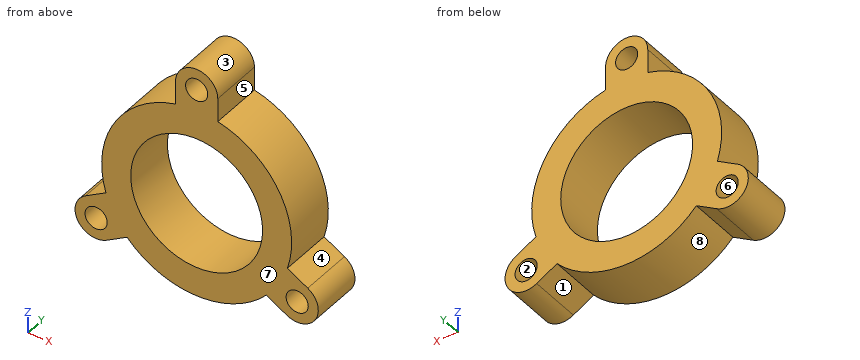
from build123d import *

# Parameters (mm, degrees)
SKETCH1_R           = 2.1
SKETCH1_R_2         = 12.5
BOSS_EXTRUDE1_DEPTH = 10


with BuildPart() as part:
    # Sketch1 → Boss-Extrude1 (new body)
    with BuildSketch(Plane(origin=(0, 0, 0), x_dir=(1, 0, 0), z_dir=(0, 1, 0))):
        with BuildLine():
            ThreePointArc((-4, -22), (0, -26), (4, -22))
            Line((4, -22), (4, -17.549928775))
            ThreePointArc((4, -17.549928775), (15.588457268, -9), (17.198684154, 5.310862772))
            Line((17.198684154, 5.310862772), (21.052558883, 7.535898385))
            ThreePointArc((21.052558883, 7.535898385), (22.516660498, 13), (17.052558883, 14.464101615))
            Line((17.052558883, 14.464101615), (13.198684154, 12.239066003))
            ThreePointArc((13.198684154, 12.239066003), (0, 18), (-13.198684154, 12.239066003))
            Line((-13.198684154, 12.239066003), (-17.052558883, 14.464101615))
            ThreePointArc((-17.052558883, 14.464101615), (-22.516660498, 13), (-21.052558883, 7.535898385))
            Line((-21.052558883, 7.535898385), (-17.198684154, 5.310862772))
            ThreePointArc((-17.198684154, 5.310862772), (-15.588457268, -9), (-4, -17.549928775))
            Line((-4, -17.549928775), (-4, -22))
        make_face()
        with Locations((0, -22)):
            Circle(SKETCH1_R, mode=Mode.SUBTRACT)
        Circle(SKETCH1_R_2, mode=Mode.SUBTRACT)
        with Locations((19.052558883, 11)):
            Circle(SKETCH1_R, mode=Mode.SUBTRACT)
        with Locations((-19.052558883, 11)):
            Circle(SKETCH1_R, mode=Mode.SUBTRACT)
    extrude(amount=BOSS_EXTRUDE1_DEPTH)


solid = part.part
Geometry: final body of the model. Coordinates: model frame, mm. Face numbers are marked on the shaded views. A direction names the side the tool comes from. Give positions to 0.01 mm unless a question says otherwise; leave off trailing zeros. Write each loop counter-clockwise with the first axis right and the second up, starting at its lowest first coordinate (ties: lowest second). Pieces come first, ordered by that corner, then holes. Notation, with made-up numbers: M -15,19.5 L 40,19.5 A17 cw 40,30.5 Z; hole C 34.25,-18.75 d5. An arc over 180 degrees is marked long. Answer in a Markdown table with one row per item. Add a question column.
(1) Ray query, line 1 (Z direction, x = 0, y = 6.5); line 2 (X direction, y = 5.75, z = -0.5); line 3 (X direction, y = 5.75, z = -11). Return the intervals inside material, ascending.
(2) First-contact query: pin 1 (5 mm diameter, centred on y = 2, z = 14, fed in from -X); pin 2 (5 mm diameter, centred on x = 18, y = 5, fed in from +Z); pin 3 (5 mm diameter, centred on y = 5.5, z = 10.5, fed in from -X). Flat tips, straight axial feed; report the tip coordinate or a pass-through.
(3) Reachability of the marked faces 1, 2, 3, 4 and 5 from +Z, -Z, +X, -X, +Y, -Y: full face, straight path, thin tool, end or side. Return the list, or none.
(4) Mould query, pull axis Z, two halves, no side actions, for the marked faces 6, 7 and 8. Classes: +Z half, -Z half, draft (parallel to the pull), parting line (faces both ways), or undercut.
(5) Section B-B on x = 0. Return loops of the section in (y, z).
(6) Section C-C on z = 0. Return loops of the section in (x, y).
(7) Section D-D on z = -11. Return loops of the section in (x, y).
(8) Section A-A on y = 6. Return loops of the section in (x, z).
Result set:
| question | item | result |
|---|---|---|
| 1 | line 1 | z = -18 to -12.5, 12.5 to 19.9, 24.1 to 26 |
| 1 | line 2 | x = -17.99 to -12.49, 12.49 to 17.99 |
| 1 | line 3 | x = -23.05 to -21.15, -16.95 to -5.94, 5.94 to 16.95, 21.15 to 23.05 |
| 2 | pin 1 | stops at x = -13.85 |
| 2 | pin 2 | stops at z = 9.15 |
| 2 | pin 3 | stops at x = -16.12 |
| 3 | face 1 | -Z, +Y, -Y |
| 3 | face 2 | +Y, -Y |
| 3 | face 3 | +Z, +Y, -Y |
| 3 | face 4 | +X, +Y, -Y |
| 3 | face 5 | +Z, +X, +Y, -Y |
| 4 | face 6 | undercut |
| 4 | face 7 | draft |
| 4 | face 8 | -Z half |
| 5 | outline | M 0,-18 L 10,-18 L 10,-12.5 L 0,-12.5 Z; M 0,12.5 L 10,12.5 L 10,19.9 L 0,19.9 Z; M 0,24.1 L 10,24.1 L 10,26 L 0,26 Z |
| 6 | outline | M -18,0 L -12.5,0 L -12.5,10 L -18,10 Z; M 12.5,0 L 18,0 L 18,10 L 12.5,10 Z |
| 7 | outline | M -23.05,0 L -21.15,0 L -21.15,10 L -23.05,10 Z; M -16.95,0 L -5.94,0 L -5.94,10 L -16.95,10 Z; M 5.94,0 L 16.95,0 L 16.95,10 L 5.94,10 Z; M 21.15,0 L 23.05,0 L 23.05,10 L 21.15,10 Z |
| 8 | outline | M -21.05,-7.54 A4 ccw -17.05,-14.46 L -13.2,-12.24 A18 ccw 13.2,-12.24 L 17.05,-14.46 A4 ccw 21.05,-7.54 L 17.2,-5.31 A18 ccw 4,17.55 L 4,22 A4 ccw -4,22 L -4,17.55 A18 ccw -17.2,-5.31 Z; hole C -19.05,-11 d4.2; hole C 0,0 d25; hole C 0,22 d4.2; hole C 19.05,-11 d4.2 |
